CAD build for the part. Positions are in the model's coordinates, mm. Face numbers are marked on the shaded views. A direction names the side the tool comes from. Round coordinates to 2 decimals unless told otherwise and drop trailing zeros. Order: outer loops, then holes, each group sorted by start corner. A loop starts at its lowest first (then second) coordinate and runs counter-clockwise, first axis right, second up. Notation, with made-up numbers: M 21.5,-17 L 30.5,-17 A5 cw 30.5,-12 Z; hole C 64.5,-12.5 d2. An arc over 180 degrees is marked long. Put each result on its own line as item: value.
```python
from build123d import *

# Parameters (mm, degrees)
SALIENTE_EXTRUIR1_DEPTH = 25
CORTAR_EXTRUIR2_REACH   = 61.582


with BuildPart() as part:
    # Croquis2 → Saliente-Extruir1 (new, symmetric)
    with BuildSketch(Plane(origin=(0, 0, 0), x_dir=(0, 0, -1), z_dir=(1, 0, 0))):
        Polygon((0, 0), (0, 45), (-15, 45), (-15, 20), (-30, 20), (-30, 0), align=None)
    extrude(amount=SALIENTE_EXTRUIR1_DEPTH, both=True)

    # Croquis4 → Cortar-Extruir2 (cut, up to next)
    with BuildSketch(Plane.XY, mode=Mode.PRIVATE) as cortar_extruir2_sk1:
        with BuildLine():
            Line((-10, 0), (10, 0))
            ThreePointArc((10, 0), (0, 10), (-10, 0))
        make_face()
    cortar_extruir2_tool1 = extrude(cortar_extruir2_sk1.sketch, amount=CORTAR_EXTRUIR2_REACH, mode=Mode.PRIVATE) & part.part
    # Croquis4 → Cortar-Extruir2 (cut, up to next)
    with BuildSketch(Plane.XY, mode=Mode.PRIVATE) as cortar_extruir2_sk2:
        Polygon((-15, 45), (-5, 30), (5, 30), (15, 45), align=None)
    cortar_extruir2_tool2 = extrude(cortar_extruir2_sk2.sketch, amount=CORTAR_EXTRUIR2_REACH, mode=Mode.PRIVATE) & part.part
    add(cortar_extruir2_tool1.solids().sort_by_distance((0, 4.244132, 0))[0], mode=Mode.SUBTRACT)
    add(cortar_extruir2_tool2.solids().sort_by_distance((0, 38.75, 0))[0], mode=Mode.SUBTRACT)


solid = part.part
```
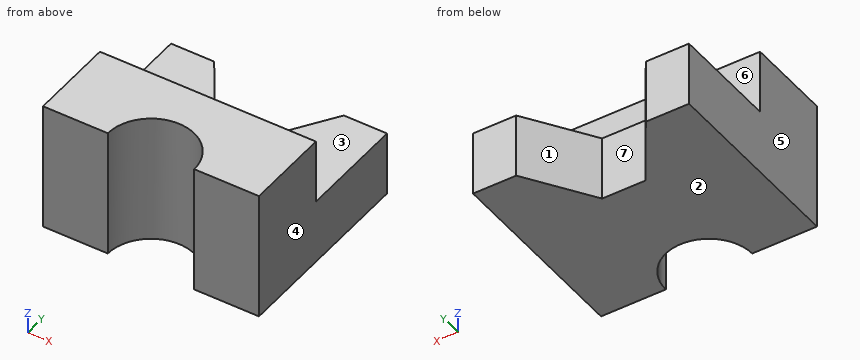
Item 1: Band-saw the part on B-B on z = 2.5. Give the cut face in (x, y).
Answers below:
outline: M -25,0 L -10,0 A10 cw 10,0 L 25,0 L 25,45 L 15,45 L 5,30 L -5,30 L -15,45 L -25,45 Z
Item 2: Band-saw the part on A-A on y = 4. Give the cut face in (x, z).
Answers below:
outline: M -25,0 L -9.17,0 L -9.17,30 L -25,30 Z; M 9.17,0 L 25,0 L 25,30 L 9.17,30 Z
Item 3: Probe line 1 along Z through (x, y) = (-20, 41); line 2 along Y through (x, z) = (16.5, 24.5); line 3 along X through (y, z) = (8, 21.5). List the from-to ranges inside material, lowest first. Write a range as [from, to].
Answers below:
line 1: [0, 15]
line 2: [0, 20]
line 3: [-25, -6], [6, 25]
Item 4: Mould opens along X. For the marked faces 4, 5, 6 and 7 say: pulls with the +X half, pulls with the -X half, needs draft (parallel to the pull), parting line crosses it, or undercut.
Answers below:
face 4: pulls with the +X half
face 5: pulls with the -X half
face 6: needs draft
face 7: undercut
Item 5: Band-saw the part on D-D on y = 41. Give the cut face in (x, z), and give its area (3 significant figures).
Answers below:
outline: M -25,0 L -12.33,0 L -12.33,15 L -25,15 Z; M 12.33,0 L 25,0 L 25,15 L 12.33,15 Z
area: 380 mm²
Item 6: Pin check, flat tips, straight feed: P1, Ø12, axis at x = 15.5, z = 24, coming from the +Y side; P2, Ø6, axis at x = 0, z = 13, coming from the -Y side; P3, Ø20, axis at x = -7.5, y = 37.5, coming from the +Z side. Stop position of each tip, or through.
Answers below:
P1: y = 20
P2: y = 9.54
P3: z = 15
Item 7: Tool access for the marked faces 1, 2 and 3: list every direction of +Z, -Z, +X, -X, +Y, -Y with a clear straight run to the whole face (end or side of a thin tool).
Answers below:
face 1: +Z, -Z, +Y
face 2: -Z, +X, -X, +Y, -Y
face 3: +Z, +X, -X, +Y
Item 8: Band-saw the part on C-C on x = 0. Give the cut face in (y, z).
Answers below:
outline: M 10,0 L 30,0 L 30,15 L 20,15 L 20,30 L 10,30 Z
